Source: three-view drawing plus pictorial views. Frame: mm from the lowest corner of the part. A direction names the side the tool comes from. Give positions to 0.01 mm unless a question says otherwise; leave off trailing zeros. Order: outer loops, then holes, each group sorted by start corner. A loop starts at its lowest first (then second) coordinate and runs counter-clockwise, first axis right, second up. Notation, with made-up numbers: (-14.75, -10.5) - (3.25, -10.5) arc R19 ccw to (3.25, 12.5) - close; hole circle Ø7 at (69.5, 5). An arc over 180 degrees is marked (long way). Answer in a Markdown table with one row per item. Add a question column.
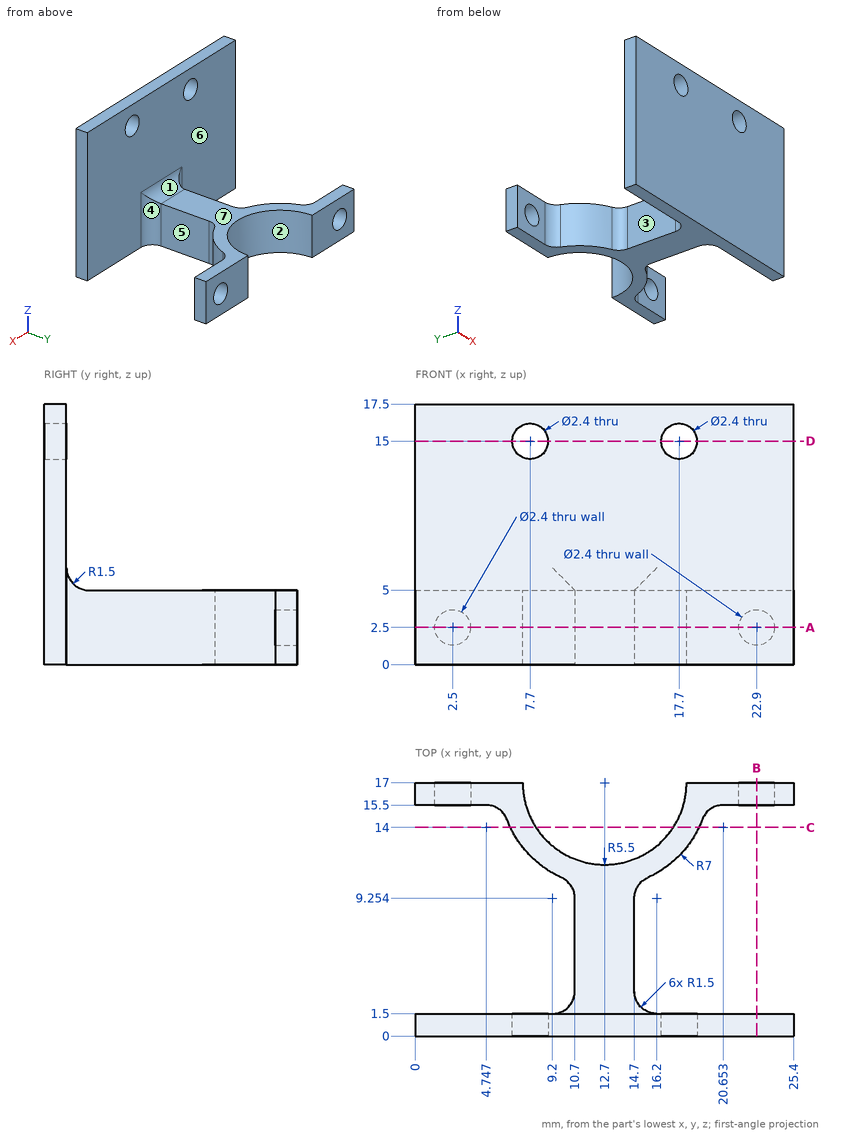
Q1. Access query for the marked faces 5, 6 and 7. Directions: +Z, -Z, +X, -X, +Y, -Y. A direction counts if a zero-diameter tool reaches every point of the face in a straight line with its end or side. Return the directions, or none.
Q2. Section D-D, the plane z = 15. Return loops of the section in (x, y), then the cut area to 3 significant figures.
Q3. Pull-direction query (X, two-part tool) for the marked faces 1, 2, 3 and 4; classes: +X half, -X half, draft (parallel to the pull), parting line (faces both ways), or undercut.
Q4. Contact query for flat-ended pins moving along their axis: P1, Ø6, axis at x = 9.5, z = 10, coming from the +Y side; P2, Ø1.4, axis at x = 17.7, z = 15, coming from the +Y side; P3, Ø4, axis at y = 4.5, z = 2.5, coming from the -X side; P4, Ø8, axis at x = 11.5, y = 12, coming from the +Z side. Output: stop coordinate, or through.
Q5. Section B-B, the plane x = 22.9. Return loops of the section in (y, z), then the cut area to 4 significant figures.
Q6. Line query: probe 1 along X at (y, z) = (0.6, 15); probe 2 along X at (y, z) = (16.1, 2.5); probe 3 along Z at (x, y) = (7.7, 1.1). Output: solid intervals per line, ascending.
Q7. Section A-A, the plane z = 2.5. State how many separate pieces and enclosed holes the cut face has, then the cut area to 3 significant figures.
Q8. Section C-C, the plane y = 14. Return loops of the section in (x, z), then the cut area to 3 significant figures.
Computed:
| question | item | result |
|---|---|---|
| 1 | face 5 | +Z, -Z, +X |
| 1 | face 6 | +Z |
| 1 | face 7 | +Z, +X, -X, +Y |
| 2 | outline | (0, 0) - (6.5, 0) - (6.5, 1.5) - (0, 1.5) - close; (8.9, 0) - (16.5, 0) - (16.5, 1.5) - (8.9, 1.5) - close; (18.9, 0) - (25.4, 0) - (25.4, 1.5) - (18.9, 1.5) - close |
| 2 | area | 30.9 mm^2 |
| 3 | face 1 | draft |
| 3 | face 2 | undercut |
| 3 | face 3 | -X half |
| 3 | face 4 | +X half |
| 4 | P1 | stops at y = 1.5 |
| 4 | P2 | passes through |
| 4 | P3 | stops at x = 10.61 |
| 4 | P4 | stops at z = 5 |
| 5 | outline | (0, 0) - (1.5, 0) - (1.5, 17.5) - (0, 17.5) - close; (15.5, 0) - (17, 0) - (17, 1.3) - (15.5, 1.3) - close; (15.5, 3.7) - (17, 3.7) - (17, 5) - (15.5, 5) - close |
| 5 | area | 30.15 mm^2 |
| 6 | probe 1 | x = 0 to 6.5, 8.9 to 16.5, 18.9 to 25.4 |
| 6 | probe 2 | x = 0 to 1.3, 3.7 to 7.27, 18.13 to 21.7, 24.1 to 25.4 |
| 6 | probe 3 | z = 0 to 13.8, 16.2 to 17.5 |
| 7 | separate pieces | 3 |
| 7 | enclosed holes | 0 |
| 7 | area | 114 mm^2 |
| 8 | outline | (6.38, 0) - (8.09, 0) - (8.09, 5) - (6.38, 5) - close; (17.31, 0) - (19.02, 0) - (19.02, 5) - (17.31, 5) - close |
| 8 | area | 17.1 mm^2 |
